CAD build for the part. Positions are in the model's coordinates, mm. A direction names the side the tool comes from. Give positions to 0.01 mm unless a question says otherwise; leave off trailing zeros. Write each loop counter-clockwise with the first axis right and the second up, starting at its lowest first coordinate (ties: lowest second). Pieces come first, ordered by that corner, then holes. Notation, with made-up numbers: (-6.75, -9.75) -> (14.25, -9.75) arc R25 ccw to (14.25, 24.25) -> close; hole circle Ø3 at (-29, -8.75). An arc over 180 degrees is marked (long way). Answer as a JSON object with one key per item and string values.
Autodesk Inventor part; units mm, degrees
ref_plane "YZ Plane" through (0, 0, 0) normal (1, 0, 0) x (0, 1, 0)
ref_plane "XZ Plane" through (0, 0, 0) normal (0, 1, 0) x (-1, 0, 0)
ref_plane "XY Plane" through (0, 0, 0) normal (0, 0, 1) x (1, 0, 0)
sketch "Sketch1" plane through (0, 0, 0) normal (0, 0, 1) x (1, 0, 0)
  line L0 (0, 0) -> (25.4, 0)
  line L1 (25.4, 0) -> (25.4, 50.8)
  line L2 (25.4, 50.8) -> (0, 50.8)
  line L3 (0, 50.8) -> (0, 0)
  dimension "d0" = 25.4
  dimension "d1" = 50.8
extrude "Extrusion1" add sketch "Sketch1" along normal blind 457.2
shell "Shell1" thickness 3.175 removed faces 2 at (8.4667, 33.8667, 0) at (8.4667, 33.8667, 457.2)
sketch "Sketch2" plane through (25.4, 0, 0) normal (1, 0, 0) x (0, 0, -1)
  line L0 (0, 50.8) -> (-457.2, 50.8)
  line L1 (-457.2, 44.45) -> (-406.4, 44.45)
  line L2 (-406.4, 44.45) -> (-406.4, 6.35)
  line L3 (-406.4, 6.35) -> (-457.2, 6.35)
  line L4 (-457.2, 6.35) -> (-457.2, 44.45)
  line L5 (0, 0) -> (0, 50.8)
  dimension "d24" = 38.1
  dimension "d26" = 6.35
  dimension "d27" = 406.4
  dimension "d28" = 50.8
extrude "Extrusion2" cut sketch "Sketch2" against normal through all
sketch "Sketch3" plane through (0, 50.8, 0) normal (0, 1, 0) x (1, 0, 0)
  line L0 (0, -457.2) -> (25.4, -457.2)
  line L1 (25.4, 0) -> (25.4, -457.2)
  line L2 (25.4, 0) -> (0, 0)
  line L3 (0, 0) -> (0, -457.2)
  circle A0 centre (12.7, -76.2) radius 3.175
  circle A1 centre (12.7, -431.8) radius 3.175
  dimension "d15" = 12.7
  dimension "d16" = 76.2
  dimension "d17" = 6.35
  dimension "d18" = 12.7
  dimension "d19" = 6.35
  dimension "d20" = 25.4
extrude "Extrusion3" cut sketch "Sketch3" against normal through all contours A0 | A1
sketch "Sketch4" plane through (25.4, 0, 0) normal (1, 0, 0) x (0, 0, -1)
  line L0 (0, 0) -> (0, 50.8)
  line L1 (0, 50.8) -> (-457.2, 50.8)
  circle A0 centre (-38.1, 38.1) radius 2.3813
  circle A1 centre (-12.7, 38.1) radius 2.3813
  circle A2 centre (-38.1, 12.7) radius 2.3813
  circle A3 centre (-12.7, 12.7) radius 2.3813
  line L2 (-38.1, 38.1) -> (-12.7, 38.1) construction
  line L3 (-12.7, 38.1) -> (-12.7, 12.7) construction
  line L4 (-12.7, 12.7) -> (-38.1, 12.7) construction
  line L5 (-38.1, 12.7) -> (-38.1, 38.1) construction
  dimension "d29" = 4.7625
  dimension "d30" = 12.7
  dimension "d31" = 25.4
  dimension "d32" = 25.4
  dimension "d33" = 12.7
extrude "Extrusion4" cut sketch "Sketch4" against normal through all
properties part number "Frame_UpperRollerMount"
1) Pin check, flat tips, straight feed: pin 1 (4 mm diameter, centred on y = 7, z = 321, fed in from -X); pin 2 (4 mm diameter, centred on x = 3, y = 39, fed in from +Z). Stop position of each tip, or through.
Model answer:
{"pin 1": "stops at x = 0", "pin 2": "stops at z = 406.4"}
2) Slice it at A-A (z = 410.5). List the corners of the cut face in (x, y) (3 decimals), then the cut area to 3 significant figures.
Model answer:
{"outline": "(0, 0) -> (25.4, 0) -> (25.4, 6.35) -> (22.225, 6.35) -> (22.225, 3.175) -> (3.175, 3.175) -> (3.175, 6.35) -> (0, 6.35) -> close; (0, 44.45) -> (3.175, 44.45) -> (3.175, 47.625) -> (22.225, 47.625) -> (22.225, 44.45) -> (25.4, 44.45) -> (25.4, 50.8) -> (0, 50.8) -> close", "area": "202 mm2"}
3) Slice it at B-B (z = 235). List the corners of the cut face in (x, y) (3 decimals), then the cut area to 3 significant figures.
Model answer:
{"outline": "(0, 0) -> (25.4, 0) -> (25.4, 50.8) -> (0, 50.8) -> close; hole (3.175, 3.175) -> (22.225, 3.175) -> (22.225, 47.625) -> (3.175, 47.625) -> close", "area": "444 mm2"}
4) 3-axis set-ups, long thin cutter, end or side, ignore diameter. For faces 4 (the flat face through (22.225, 25, 225)), 5 (the flat face through (0, 26, 225)): which of +Z, -Z, +X, -X, +Y, -Y reach the whole face in a straight line?
Model answer:
{"face 4": "+Z, -Z", "face 5": "+Z, -Z, -X, +Y, -Y"}
5) Mould opens along Y. For faces 1 (the flat face through (3.175, 26, 225)), 2 (the flat face through (13, 0, 225)), 3 (the flat face through (13, 50.8, 225)) say: released by +Y, released by -Y, zero draft, split by the parting line, or undercut.
Model answer:
{"face 1": "undercut", "face 2": "released by -Y", "face 3": "released by +Y"}
6) Slice it at C-C (y = 24.5). List the corners of the cut face in (x, z) (3 decimals), then the cut area to 3 significant figures.
Model answer:
{"outline": "(0, 0) -> (3.175, 0) -> (3.175, 406.4) -> (0, 406.4) -> close; (22.225, 0) -> (25.4, 0) -> (25.4, 406.4) -> (22.225, 406.4) -> close", "area": "2,580 mm2"}
7) Wall check: probe 1 along Y at (x, z) = (0.9, 38.1); probe 2 along Z at (x, y) = (12.7, 48.6) (3 decimals); probe 3 along X at (y, z) = (25, 373) (3 decimals). Give the ranges that are in metal, low to high.
Model answer:
{"probe 1": "y = 0 to 10.32, 15.08 to 35.72, 40.48 to 50.8", "probe 2": "z = 0 to 73.025, 79.375 to 428.625, 434.975 to 457.2", "probe 3": "x = 0 to 3.175, 22.225 to 25.4"}
